The listing builds one solid part. Answer for the finished solid, in the listing's coordinates (mm). A direction names the side the tool comes from. Round coordinates to 2 decimals unless told otherwise and drop trailing zeros. Write each loop counter-clockwise with the first axis right and the second up, starting at its lowest first coordinate (ties: lowest second). Pieces come first, ordered by that corner, then holes. Notation, with made-up numbers: (-24, 4.25) - (-4, 4.25) arc R37 cw to (-4, 40.25) - close; hole circle Ø7 at (35, 24). An arc over 180 degrees is marked (long way). Answer as CSV lines item,"result". Start each with the question number.
Item 1: Which of the six approach directions +Z, -Z, +X, -X, +Y, -Y give full straight-line access (tool end or side, diameter ignored) to faces 1 (the flat face through (-1, -10, 45.769)), 2 (the flat face through (41, -53, 25.769))?
Item 2: A cutting plane is placed at C-C on x = 27. Determine the outline of the cut face in (y, z).
Item 3: A cutting plane is placed at A-A on z = 31. Determine the outline of the cut face in (x, y), and give its area (3 significant figures).
Item 4: Straight lines are drawn through the part: line 1 along X through (y, z) = (-46, 9); line 2 along Z through (x, y) = (32, -27); line 3 along Z through (x, y) = (28, -38). For each, find the intervals that lie inside material, in ascending order. Write a range as [from, to].
Item 5: A cutting plane is placed at D-D on y = -35.5. Determine the outline of the cut face in (x, z).
Item 6: A cutting plane is placed at B-B on x = -39.5. Determine the outline of the cut face in (y, z), and give its area (3 significant figures).
Item 7: Flat-ended cylindrical pins translate along their axes: pin 1 (3.5 mm diameter, centred on x = 41, y = -54, fed in from +Z); pin 2 (21.5 mm diameter, centred on x = -30.5, y = -48.5, fed in from +Z). Find the tip coordinate at first contact, or state that the pin passes through.
```python
from build123d import *

# Parameters (mm, degrees)
F0_W        = 93.9634628594
F0_H        = 91.5375761688
F1_DEPTH    = 40
F2_R        = 14.2987523314
F3_DEPTH    = 64.5675584674
F4_T1_DEPTH = 193.9634628594
F6_DEPTH    = 26.9540566951


# Not quite as in the source:
# - a fillet or chamfer that OpenCascade refuses, or shapes differently, is made with other operations: its cross-section is extruded or revolved along the edge and cut away or added


with BuildPart() as f1:
    # F0 (on Front) → F1 (new body)
    with BuildSketch(Plane.XZ):
        Rectangle(F0_W, F0_H)
    extrude(amount=F1_DEPTH)

    # F2 (on face) → F3 (cut)
    with BuildSketch(Plane.XZ.offset(40)):
        with Locations((23.1474172324, 18.2785931975)):
            Circle(F2_R)
    extrude(amount=-F3_DEPTH, mode=Mode.SUBTRACT)

    # F4: fillet of radius 20 on 1 edges, made by hand

    # F4_s2 → F4_t1 (cut)
    with BuildSketch(Plane.YZ.offset(-96.9817314297)):
        with BuildLine():
            ThreePointArc((-20, 45.7687880844), (-34.1421356237, 39.9109237081), (-40, 25.7687880844))
            Line((-40, 25.7687880844), (-40, 45.7687880844))
            Line((-40, 45.7687880844), (-20, 45.7687880844))
        make_face()
    extrude(amount=F4_T1_DEPTH, mode=Mode.SUBTRACT)

    # F5 (on face) → F6 (join)
    with BuildSketch(Plane.XZ.offset(40)):
        with BuildLine():
            Line((-46.9817314297, 25.7687880844), (-46.9817314297, -45.7687880844))
            Line((-46.9817314297, -45.7687880844), (46.9817314297, -45.7687880844))
            Line((46.9817314297, -45.7687880844), (46.9817314297, 25.7687880844))
            Line((46.9817314297, 25.7687880844), (35.3273720267, 25.7687880844))
            ThreePointArc((35.3273720267, 25.7687880844), (36.9062775639, 22.1706467187), (37.4461695638, 18.2785931975))
            ThreePointArc((37.4461695638, 18.2785931975), (19.2553637112, 4.5197328659), (10.9674624381, 25.7687880844))
            Line((10.9674624381, 25.7687880844), (-46.9817314297, 25.7687880844))
        make_face()
    extrude(amount=F6_DEPTH)


solid = f1.part
```
Geometry says:
1,face 1,"+Z, +X, -X, +Y, -Y"
1,face 2,"+Z, +X, -X, -Y"
2,outline,"(-66.95, -45.77) - (0, -45.77) - (0, 4.51) - (-66.95, 4.51) - close; (-38.99, 32.05) - (0, 32.05) - (0, 45.77) - (-20, 45.77) arc R20 ccw to start"
3,outline,"(-46.98, -39.3) - (16.62, -39.3) - (16.62, 0) - (-46.98, 0) - close; (29.68, -39.3) - (46.98, -39.3) - (46.98, 0) - (29.68, 0) - close"
3,area,"3,180 mm^2"
4,line 1,"x = [-46.98, 12.27], [34.03, 46.98]"
4,line 2,"z = [-45.77, 7.05], [29.51, 44.5]"
4,line 3,"z = [-45.77, 4.83], [31.73, 34.49]"
5,outline,"(-46.98, -45.77) - (46.98, -45.77) - (46.98, 38.41) - (-46.98, 38.41) - close; hole circle Ø28.6 at (23.15, 18.28)"
6,outline,"(-66.95, -45.77) - (0, -45.77) - (0, 45.77) - (-20, 45.77) arc R20 ccw to (-40, 25.77) - (-66.95, 25.77) - close"
6,area,"5,500 mm^2"
7,pin 1,"stops at z = 25.77"
7,pin 2,"stops at z = 34.98"
